```python
from build123d import *

# Parameters (mm, degrees)
F0_R     = 2.6
F1_DEPTH = 5.3
F2_R     = 7.25
F3_DEPTH = 6
F2_R_2   = 2.6
F4_DEPTH = 2.7
F5_W     = 12
F5_H     = 6.2
F6_DEPTH = 2
F7_R     = 3.7
F8_DEPTH = 19


with BuildPart() as f1:
    # F0 (on Top) → F1 (new body)
    with BuildSketch(Plane.XY):
        with BuildLine():
            Line((-16.354793, -5.071878), (-16.354793, -0.071878))
            Line((-16.354793, -0.071878), (-16.354793, 4.928122))
            Line((-16.354793, 4.928122), (-31.283726, 4.928122))
            ThreePointArc((-31.283726, 4.928122), (-33.197143, 5.308724), (-34.819259, 6.392588))
            Line((-34.819259, 6.392588), (-36.324322, 7.89765))
            ThreePointArc((-36.324322, 7.89765), (-37.454863, 8.745723), (-38.77755, 9.243572))
            Line((-38.77755, 9.243572), (-50.703144, 11.887689))
            ThreePointArc((-50.703144, 11.887689), (-65.604793, -0.071878), (-50.703144, -12.031446))
            Line((-50.703144, -12.031446), (-38.77755, -9.387329))
            ThreePointArc((-38.77755, -9.387329), (-37.454863, -8.88948), (-36.324322, -8.041406))
            Line((-36.324322, -8.041406), (-34.819259, -6.536344))
            ThreePointArc((-34.819259, -6.536344), (-33.197143, -5.45248), (-31.283726, -5.071878))
            Line((-31.283726, -5.071878), (-16.354793, -5.071878))
        make_face()
        with Locations((-32.854793, -0.071878)):
            Circle(F0_R, mode=Mode.SUBTRACT)
    extrude(amount=F1_DEPTH)

    # F2 (on face) → F3 (join)
    with BuildSketch(Plane.XY.offset(5.3)):
        with Locations((-53.354793, -0.071878)):
            Circle(F2_R)
    extrude(amount=F3_DEPTH)

    # F2 (on face) → F4 (join)
    with BuildSketch(Plane.XY.offset(5.3)):
        with BuildLine():
            ThreePointArc((-46.454594, 10.94571), (-40.354793, -0.071878), (-46.454594, -11.089466))
            Line((-46.454594, -11.089466), (-38.77755, -9.387329))
            ThreePointArc((-38.77755, -9.387329), (-37.454863, -8.88948), (-36.324322, -8.041406))
            Line((-36.324322, -8.041406), (-34.819259, -6.536344))
            ThreePointArc((-34.819259, -6.536344), (-33.197143, -5.45248), (-31.283726, -5.071878))
            Line((-31.283726, -5.071878), (-16.354793, -5.071878))
            Line((-16.354793, -5.071878), (-16.354793, -0.071878))
            Line((-16.354793, -0.071878), (-16.354793, 4.928122))
            Line((-16.354793, 4.928122), (-31.283726, 4.928122))
            ThreePointArc((-31.283726, 4.928122), (-33.197143, 5.308724), (-34.819259, 6.392588))
            Line((-34.819259, 6.392588), (-36.324322, 7.89765))
            ThreePointArc((-36.324322, 7.89765), (-37.454863, 8.745723), (-38.77755, 9.243572))
            Line((-38.77755, 9.243572), (-46.454594, 10.94571))
        make_face()
        with Locations((-32.854793, -0.071878)):
            Circle(F2_R_2, mode=Mode.SUBTRACT)
    extrude(amount=F4_DEPTH)

    # F5 (on face) → F6 (join)
    with BuildSketch(Plane.XY.offset(8)):
        with Locations((-22.354793, -0.071878)):
            Rectangle(F5_W, F5_H)
    extrude(amount=F6_DEPTH)

    # F7 (on face) → F8 (join)
    with BuildSketch(Plane.XY.offset(11.3)):
        with Locations((-53.354793, -0.071878)):
            Circle(F7_R)
    extrude(amount=F8_DEPTH)


solid = f1.part
```
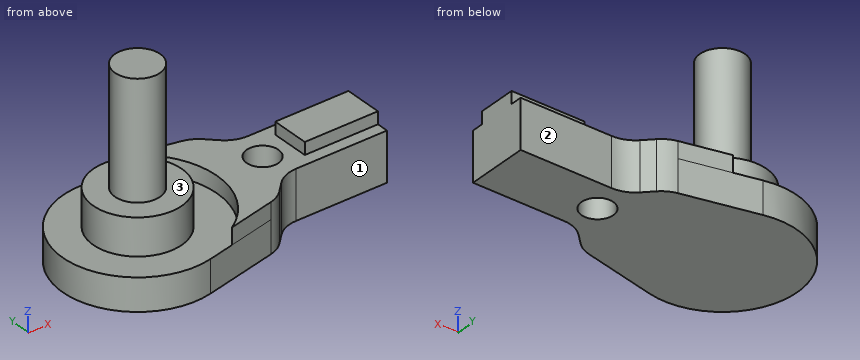
The model under review builds one solid part; all positions refer to its coordinate system, in mm. Face numbers are marked on the shaded views. A direction names the side the tool comes from. Round coordinates to 2 decimals unless told otherwise and drop trailing zeros. Loops run counter-clockwise (first coordinate to the right, second up) from the corner with the lowest first, then second, coordinate; pieces in that order, holes last. Notation, with made-up numbers: M 58,55.25 L 116,55.25 A34 cw 116,94.25 Z; hole C -36,19.5 d2. An arc over 180 degrees is marked long. Write item = value, one per line.
Item 1: For line 1 (Z direction, x = -28.5, y = -3.75); line 2 (Y direction, x = -20, z = 6.5); line 3 (X direction, y = 2, z = 9), list the stretches that pass through material, from the lowest coordinate up. Write a range as [from, to].
Return value:
line_1 = [0, 8]
line_2 = [-5.07, 4.93]
line_3 = [-60.3, -46.41], [-28.35, -16.35]
Item 2: Take a section at D-D on z = 28. Write out the cut boundary in (x, y), then the cut area to 3 significant figures.
Return value:
outline = C -53.35,-0.07 d7.4
area = 43.0 mm2
Item 3: Machinability: for the marked faces 1, 2 and 3, which of the approach directions +Z, -Z, +X, -X, +Y, -Y give a long, thin tool a straight path to every point of the face, cutting with its end or side? Answer none if there is none.
Return value:
face_1 = +Z, -Z, +X, -Y
face_2 = +Z, -Z, +X, +Y
face_3 = +Z
Item 4: Take a section at C-C on x = -27. Write out the cut boundary in (y, z).
Return value:
outline = M -5.07,0 L 4.93,0 L 4.93,8 L 3.03,8 L 3.03,10 L -3.17,10 L -3.17,8 L -5.07,8 Z
Item 5: Insertion check: P1, Ø9, axis at x = -23, z = 5.5, coming from the -Y side; P2, Ø10, axis at y = -9.5, z = 6.5, coming from the -X side; P3, Ø0.6, axis at y = -0.5, z = 9.5, coming from the -X side. Each pin has a flat end and moves straight along its axis. Give the tip position at first contact, or say it passes through.
Return value:
P1 = -5.07
P2 = -64.72
P3 = -60.6
Item 6: Take a section at B-B on z = 3. Write out the cut boundary in (x, y), then the cut area to 3 significant figures.
Return value:
outline = M -50.7,-12.03 L -38.78,-9.39 A5 ccw -36.32,-8.04 L -34.82,-6.54 A5 cw -31.28,-5.07 L -16.35,-5.07 L -16.35,4.93 L -31.28,4.93 A5 cw -34.82,6.39 L -36.32,7.9 A5 ccw -38.78,9.24 L -50.7,11.89 A12.25 ccw long Z; hole C -32.85,-0.07 d5.2
area = 785 mm2
Item 7: Take a section at A-A on y = 1.25. Write out the cut boundary in (x, z).
Return value:
outline = M -65.53,0 L -35.09,0 L -35.09,8 L -40.42,8 L -40.42,5.3 L -46.23,5.3 L -46.23,11.3 L -49.9,11.3 L -49.9,30.3 L -56.81,30.3 L -56.81,11.3 L -60.48,11.3 L -60.48,5.3 L -65.53,5.3 Z; M -30.62,0 L -16.35,0 L -16.35,10 L -28.35,10 L -28.35,8 L -30.62,8 Z
